```python
from build123d import *

# Parameters (mm, degrees)
SKETCH2_R          = 1.125
CUT_EXTRUDE1_DEPTH = 9.5875
SKETCH3_R          = 1.125
CUT_EXTRUDE2_DEPTH = 9.5875
CIRPATTERN1_COUNT  = 4


with BuildPart() as part:
    # Sketch1 → Revolve1 (revolve)
    with BuildSketch(Plane.XY):
        Polygon((-23.5, 8.5875), (-18.65, 8.5875), (-18.65, 1.5875), (-16.11, 1.5875), (-16.11, 0), (-23.5, 0), align=None)
    revolve(axis=Axis((0, 0, 0), (0, 1, 0)))

    # Sketch2 → Cut-Extrude1 (cut, through all)
    with BuildSketch(Plane(origin=(0, 0, 0), x_dir=(-1, 0, 0), z_dir=(0, -1, 0))):
        with Locations((19.177, 0)):
            Circle(SKETCH2_R)
    cut_extrude1 = extrude(amount=-CUT_EXTRUDE1_DEPTH, mode=Mode.SUBTRACT)

    # Sketch3 → Cut-Extrude2 (cut, through all)
    with BuildSketch(Plane.XZ):
        with Locations((-14.495689029, 14.495689029)):
            Circle(SKETCH3_R)
    cut_extrude2 = extrude(amount=-CUT_EXTRUDE2_DEPTH, mode=Mode.SUBTRACT)

    # CirPattern1: Cut-Extrude1, Cut-Extrude2 ×4 about axis
    cirpattern1_axis = Axis((0, 0, 0), (0, 1, 0))
    for i in range(1, CIRPATTERN1_COUNT):
        add(cut_extrude1.rotate(cirpattern1_axis, i * 360 / CIRPATTERN1_COUNT), mode=Mode.SUBTRACT)
        add(cut_extrude2.rotate(cirpattern1_axis, i * 360 / CIRPATTERN1_COUNT), mode=Mode.SUBTRACT)


solid = part.part
```
Read the model definition and answer for the solid it produces. Units are mm, in the model's axes. A direction names the side the tool comes from. Give positions to 0.01 mm unless a question says otherwise; leave off trailing zeros. Write each loop counter-clockwise with the first axis right and the second up, starting at its lowest first coordinate (ties: lowest second). Pieces come first, ordered by that corner, then holes. Notation, with made-up numbers: (16, 3) -> (40, 3) arc R30 ccw to (40, 25) -> close; hole circle Ø8 at (27.25, 45). An arc over 180 degrees is marked (long way). Answer in a Markdown table with one row per item.
1) Determine the mould class of faces 1 (the flat face through (-5.6, 0, -15.3)), 2 (the cylindrical face through (-13.42, 4.23, 14.83)), 3 (the cylindrical face through (-22.4, 4.4, 7.1)), 4 (the cylindrical face through (16.094, 0.783, 0.708)) for opening direction X: released by +X, released by -X, zero draft, split by the parting line, or undercut.
Results list:
| item | result |
|---|---|
| face 1 | zero draft |
| face 2 | undercut |
| face 3 | split by the parting line |
| face 4 | undercut |
2) A tool of negligible diameter and unlimited length cuts with its end or side. For faces 5 (the cylindrical face through (20.216, 4.234, -0.431)), 6 (the cylindrical face through (-13.322, 5.039, 13.052)), from which of +Z, -Z, +X, -X, +Y, -Y can it reach the whole face along a straight path? Write none if from no direction.
Results list:
| item | result |
|---|---|
| face 5 | +Y, -Y |
| face 6 | +Y |
3) Each of these flat-tipped pins is pushed along its axis until it touches: pin 1 Ø4 at (x, z) = (-14, -1) entering from +Y; pin 2 Ø2 at (y, z) = (5.5, -15.5) entering from +X; pin 3 Ø4 at (x, y) = (10, 6) entering from -Z; pin 4 Ø4 at (y, z) = (1.5, 9.5) entering from -X. Where does it stop, or does it pass through?
Results list:
| item | result |
|---|---|
| pin 1 | through |
| pin 2 | x = 18.49 |
| pin 3 | z = -22.1 |
| pin 4 | x = -22.27 |
4) Straight lines are drawn through the part: line 1 (Z direction, x = -15, y = 5.75); line 2 (Z direction, x = 9, y = 2.5); line 3 (Z direction, x = 20, y = 2). For each, find the intervals that lie inside material, in ascending order. Write a range as [from, to].
Results list:
| item | result |
|---|---|
| line 1 | [-18.09, -15.5], [-13.49, -11.08], [11.08, 13.49], [15.5, 18.09] |
| line 2 | [-21.71, -16.33], [16.33, 21.71] |
| line 3 | [-12.34, -0.77], [0.77, 12.34] |
5) Section A-A on z = 0 is taken. Give the vertices of the cut face in (x, y).
Results list:
| item | result |
|---|---|
| outline | (-23.5, 0) -> (-20.3, 0) -> (-20.3, 8.59) -> (-23.5, 8.59) -> close; (-18.05, 0) -> (-16.11, 0) -> (-16.11, 1.59) -> (-18.05, 1.59) -> close; (16.11, 0) -> (18.05, 0) -> (18.05, 1.59) -> (16.11, 1.59) -> close; (20.3, 0) -> (23.5, 0) -> (23.5, 8.59) -> (20.3, 8.59) -> close |
6) Section C-C on x = 10 is taken. Give the vertices of the cut face in (y, z).
Results list:
| item | result |
|---|---|
| outline | (0, -21.27) -> (8.59, -21.27) -> (8.59, -15.74) -> (1.59, -15.74) -> (1.59, -12.63) -> (0, -12.63) -> close; (0, 12.63) -> (1.59, 12.63) -> (1.59, 15.74) -> (8.59, 15.74) -> (8.59, 21.27) -> (0, 21.27) -> close |
7) Section B-B on x = 0 is taken. Give the vertices of the cut face in (y, z), plus the area to 3 significant figures.
Results list:
| item | result |
|---|---|
| outline | (0, -23.5) -> (8.59, -23.5) -> (8.59, -20.3) -> (0, -20.3) -> close; (0, -18.05) -> (1.59, -18.05) -> (1.59, -16.11) -> (0, -16.11) -> close; (0, 16.11) -> (1.59, 16.11) -> (1.59, 18.05) -> (0, 18.05) -> close; (0, 20.3) -> (8.59, 20.3) -> (8.59, 23.5) -> (0, 23.5) -> close |
| area | 61.1 mm^2 |
8) Section D-D on y = 3.75 is taken. Give the vertices of the cut face in (x, z) (3 decimals).
Results list:
| item | result |
|---|---|
| outline | circle Ø47 at (0, 0); hole (-18.624, -0.98) arc R18.65 ccw to (-0.98, -18.624) arc R1.125 ccw (long way) to (0.98, -18.624) arc R18.65 ccw to (18.624, -0.98) arc R1.125 ccw (long way) to (18.624, 0.98) arc R18.65 ccw to (0.98, 18.624) arc R1.125 ccw (long way) to (-0.98, 18.624) arc R18.65 ccw to (-18.624, 0.98) arc R1.125 ccw (long way) to start; hole circle Ø2.25 at (-14.496, -14.496); hole circle Ø2.25 at (-14.496, 14.496); hole circle Ø2.25 at (14.496, -14.496); hole circle Ø2.25 at (14.496, 14.496) |
